Can you work these out from the model? Positions are in its coordinate system, mm. Face numbers are marked on the shaded views. A direction names the side the tool comes from. Coordinates: 2 decimals unless noted, no trailing zeros. Loops run counter-clockwise (first coordinate to the right, second up) from the corner with the lowest first, then second, coordinate; pieces in that order, holes last. Notation, with made-up numbers: M 17.5,89.5 L 27.5,89.5 A34 cw 27.5,125.5 Z; hole C 63.25,54 d1. An arc over 180 degrees is marked long. Answer as a JSON object with one key per item and string values. Group by question number.
Item 1: I'm going to push flat-ended pins straight in: pin 1 Ø6 at (y, z) = (-41.5, 12.5) entering from -X; pin 2 Ø9.5 at (x, y) = (-7.5, -6) entering from +Z; pin 3 Ø8 at (y, z) = (-97, 3.5) entering from +X; pin 4 Ø3 at (x, y) = (9, -50) entering from +Z. Where does each tip first touch, or does it pass through?
Item 2: If I drill on line 1 (X direction, y = -154, z = 17.5); line 2 (Y direction, x = -14, z = 2.5); line 3 (Y direction, x = 6, z = 21.5), over which ranges is the centre line in solid material (lowest first)?
Item 3: Suppose I cut it at D-D (z = 4.5). Write out the boundary of the cut face in (x, y), then the cut area to 3 significant figures.
Item 4: Suppose I cut it at C-C (y = 0). Write out the boundary of the cut face in (x, z).
Item 5: Which directions (+Z, -Z, +X, -X, +Y, -Y) give clear straight access to the entire face, cutting with the end or side of a thin tool? Please do the marked faces 1 and 2.
Item 6: Suppose I cut it at A-A (x = 0). Write out the boundary of the cut face in (y, z).
Item 7: We'd pull the mould along Y, two halves only. Please class the marked faces 3, 4 and 5: +Y half, -Y half, draft (parallel to the pull), parting line (faces both ways), or undercut.
Item 8: Suppose I cut it at B-B (z = 18). Write out the boundary of the cut face in (x, y), then the cut area to 3 significant figures.
```python
from build123d import *

# Parameters (mm, degrees)
BOSS_EXTRUDE1_DEPTH = 7.5
SKETCH7_W           = 100
SKETCH7_H           = 35
BOSS_EXTRUDE2_DEPTH = 8
SKETCH5_R           = 16.1
CUT_EXTRUDE1_DEPTH  = 10
SKETCH6_R           = 10
CUT_EXTRUDE2_DEPTH  = 20
SKETCH11_R          = 1.4
CUT_EXTRUDE3_DEPTH  = 8
SKETCH12_R          = 1.4
CUT_EXTRUDE4_DEPTH  = 8


with BuildPart() as part:
    # Sketch1 → Boss-Extrude1 (new, symmetric)
    with BuildSketch(Plane.XY):
        with BuildLine():
            Line((24.668742494, 4.056247498), (50, -150))
            Line((50, -150), (-50, -150))
            Line((-50, -150), (-24.668742494, 4.056247498))
            ThreePointArc((-24.668742494, 4.056247498), (0, 25), (24.668742494, 4.056247498))
        make_face()
    extrude(amount=BOSS_EXTRUDE1_DEPTH, both=True)

    # Sketch7 → Boss-Extrude2 (add)
    with BuildSketch(Plane.XZ.offset(150)):
        with Locations((0, 10)):
            Rectangle(SKETCH7_W, SKETCH7_H)
    extrude(amount=BOSS_EXTRUDE2_DEPTH)

    # Sketch5 → Cut-Extrude1 (cut)
    with BuildSketch(Plane.XY.offset(7.5)):
        Circle(SKETCH5_R)
    extrude(amount=-CUT_EXTRUDE1_DEPTH, mode=Mode.SUBTRACT)

    # Sketch6 → Cut-Extrude2 (cut)
    with BuildSketch(Plane.XY.offset(-2.5)):
        Circle(SKETCH6_R)
    extrude(amount=-CUT_EXTRUDE2_DEPTH, mode=Mode.SUBTRACT)

    # Sketch10 → M5 Clearance Hole1 (revolve, cut)
    with BuildSketch(Plane(origin=(-30, -150, 17.5), x_dir=(0, 0, 1), z_dir=(1, 0, 0))):
        Polygon((0, 0), (0, 11.652366702), (2.75, 10), (2.75, 0), align=None)
    m5_clearance_hole1 = revolve(axis=Axis((-30, -143.65, 17.5), (0, -1, 0)), mode=Mode.SUBTRACT)

    # Mirror1: M5 Clearance Hole1 across plane
    add(m5_clearance_hole1.mirror(Plane(origin=(0, 0, 0), x_dir=(0, 0, 1), z_dir=(1, 0, 0))), mode=Mode.SUBTRACT)

    # Sketch11 → Cut-Extrude3 (cut)
    with BuildSketch(Plane.XY.offset(7.5)):
        with Locations((14, 14.282856857)):
            Circle(SKETCH11_R)
        with Locations((-14, 14.282856857)):
            Circle(SKETCH11_R)
    extrude(amount=-CUT_EXTRUDE3_DEPTH, mode=Mode.SUBTRACT)

    # Sketch12 → Cut-Extrude4 (cut)
    with BuildSketch(Plane(origin=(0, 0, -7.5), x_dir=(-1, 0, 0), z_dir=(0, 0, -1))):
        with Locations((9, -50)):
            Circle(SKETCH12_R)
        with Locations((-9, -50)):
            Circle(SKETCH12_R)
    extrude(amount=-CUT_EXTRUDE4_DEPTH, mode=Mode.SUBTRACT)


solid = part.part
```
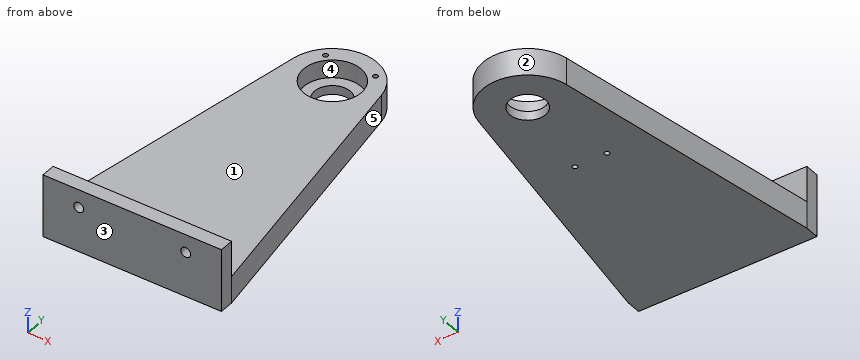
From the geometry:
{
 "1": {"pin 1": "through", "pin 2": "z = -2.5", "pin 3": "x = 41.94", "pin 4": "z = 7.5"},
 "2": {"line 1": "-50 to -32.75, -27.25 to 27.25, 32.75 to 50", "line 2": "-158 to -7.95, 7.95 to 12.88, 15.68 to 20.71", "line 3": "-158 to -150"},
 "3": {"outline": "M -50,-158 L 50,-158 L 50,-150 L 24.67,4.06 A25 ccw -24.67,4.06 L -50,-150 Z; hole C 0,0 d32.2; hole C -14,14.28 d2.8; hole C 14,14.28 d2.8", "area": "12,300 mm2"},
 "4": {"outline": "M -25.34,-7.5 L -10,-7.5 L -10,-2.5 L -16.1,-2.5 L -16.1,7.5 L -25.34,7.5 Z; M 10,-7.5 L 25.34,-7.5 L 25.34,7.5 L 16.1,7.5 L 16.1,-2.5 L 10,-2.5 Z"},
 "5": {"face 1": "+Z, +X, -X, +Y", "face 2": "+Z, -Z, +Y"},
 "6": {"outline": "M -158,-7.5 L -10,-7.5 L -10,-2.5 L -16.1,-2.5 L -16.1,7.5 L -150,7.5 L -150,27.5 L -158,27.5 Z; M 10,-7.5 L 25,-7.5 L 25,7.5 L 16.1,7.5 L 16.1,-2.5 L 10,-2.5 Z"},
 "7": {"face 3": "-Y half", "face 4": "undercut", "face 5": "+Y half"},
 "8": {"outline": "M -50,-158 L -32.7,-158 L -32.7,-150 L -50,-150 Z; M -27.3,-158 L 27.3,-158 L 27.3,-150 L -27.3,-150 Z; M 32.7,-158 L 50,-158 L 50,-150 L 32.7,-150 Z", "area": "713 mm2"}
}
